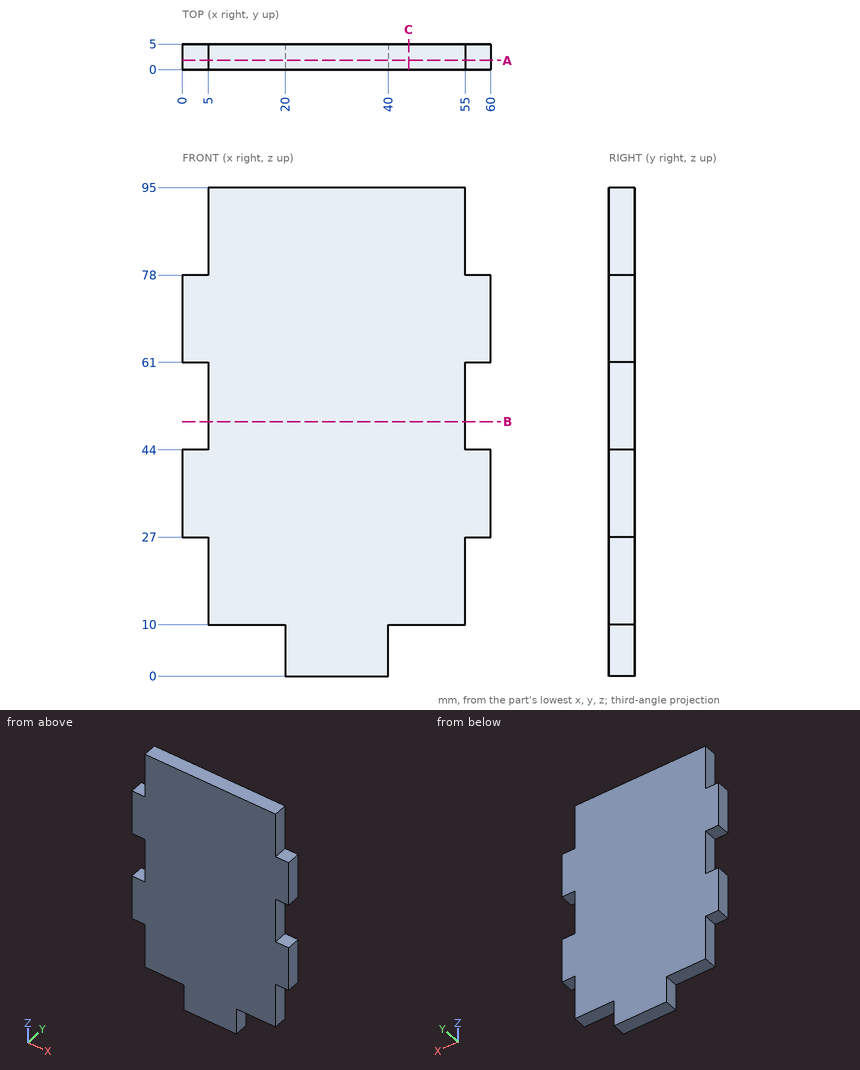
Input: dimensioned drawing with shaded views. Units: mm. Origin: part minimum x, y, z. Give positions to 0.01 mm unless a question says otherwise; leave off trailing zeros. Write each loop counter-clockwise with the first axis right and the second up, starting at its lowest first coordinate (ties: lowest second). Pieces come first, ordered by that corner, then holes.
1. Section query A-A (y = 1.8). Return the cut outline in (x, z).
2. Section query C-C (x = 44). Return the cut outline in (y, z), then the cut area to 3 significant figures.
3. First-contact query: pin 1 (2 mm diameter, centred on x = 48.5, z = 15.5, fed in from -Y); pin 2 (1.5 mm diameter, centred on x = 10.5, y = 3.5, fed in from -Z); pin 3 (2.5 mm diameter, centred on y = 2.5, z = 21.5, fed in from +X); pin 4 (1.5 mm diameter, centred on x = 3, y = 3, fed in from -Z). Flat tips, straight axial feed; report the tip coordinate or a pass-through.
4. Section query B-B (z = 49.5). Return the cut outline in (x, y), then the cut area to 3 significant figures.
5. Material intervals for line 1 along X through (y, z) = (2.75, 48.5); line 2 along Z through (x, y) = (14, 3.6), sorted ascending.
Output values:
1. outline: (0, 27) - (5, 27) - (5, 10) - (20, 10) - (20, 0) - (40, 0) - (40, 10) - (55, 10) - (55, 27) - (60, 27) - (60, 44) - (55, 44) - (55, 61) - (60, 61) - (60, 78) - (55, 78) - (55, 95) - (5, 95) - (5, 78) - (0, 78) - (0, 61) - (5, 61) - (5, 44) - (0, 44) - close
2. outline: (0, 10) - (5, 10) - (5, 95) - (0, 95) - close
2. area: 425 mm2
3. pin 1: stops at y = 0
3. pin 2: stops at z = 10
3. pin 3: stops at x = 55
3. pin 4: stops at z = 27
4. outline: (5, 0) - (55, 0) - (55, 5) - (5, 5) - close
4. area: 250 mm2
5. line 1: x = 5 to 55
5. line 2: z = 10 to 95
